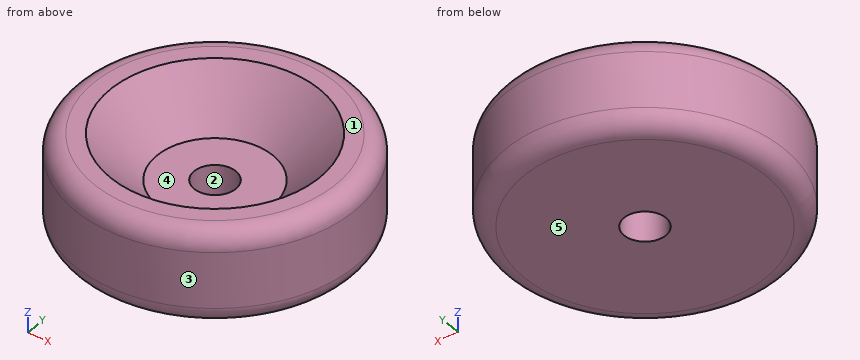
from build123d import *

# Parameters (mm, degrees)
F0_R     = 15
F0_R_2   = 11
F0_R_3   = 4.25
F1_DEPTH = 10
F2_R     = 2
F0_R_4   = 2.25
F3_DEPTH = 5


# Not quite as in the source:
# - a fillet or chamfer that OpenCascade refuses, or shapes differently, is made with other operations: its cross-section is extruded or revolved along the edge and cut away or added


with BuildPart() as f1:
    # F0 (on Top) → F1 (new body)
    with BuildSketch(Plane.XY):
        Circle(F0_R)
        Circle(F0_R_2, mode=Mode.SUBTRACT)
        Circle(F0_R_2)
        Circle(F0_R_3, mode=Mode.SUBTRACT)
    extrude(amount=F1_DEPTH)

    # F2
    f2_edges = [f1.edges().sort_by_distance(p)[0] for p in [
        (-15, 0, 10),
        (15, 0, 5),
        (-15, 0, 0),
    ]]
    fillet(f2_edges, radius=F2_R)

    # F0 (on Top) → F3 (join)
    with BuildSketch(Plane.XY):
        Circle(F0_R_3)
        Circle(F0_R_4, mode=Mode.SUBTRACT)
    extrude(amount=F3_DEPTH)

    # F4: chamfer of 7 on 1 edges, made by hand


with BuildPart() as f4_tool2:
    # F4_s3 → F4_t4 (revolve)
    with BuildSketch(Plane.XZ):
        Polygon((11.25, 10), (4.25, 3), (4.25, 10), align=None)
    revolve(axis=Axis((0, 0, 10), (0, 0, 1)))

    split(bisect_by=Plane.XY.offset(5), keep=Keep.TOP)


with BuildPart() as f1_1:
    add(f1.part)

    # F4_t1: cut F4_tool2
    add(f4_tool2.part, mode=Mode.SUBTRACT)


solid = f1_1.part
CAD build for the part. Positions are in the model's coordinates, mm. Face numbers are marked on the shaded views. A direction names the side the tool comes from. Give positions to 0.01 mm unless a question says otherwise; leave off trailing zeros. Write each loop counter-clockwise with the first axis right and the second up, starting at its lowest first coordinate (ties: lowest second). Pieces come first, ordered by that corner, then holes. Notation, with made-up numbers: (19.25, 78.5) -> (39.25, 78.5) arc R7 ccw to (39.25, 85.5) -> close; hole circle Ø11 at (57, 43). An arc over 180 degrees is marked (long way). Return JSON: item names as keys, results as strings.
Item 1: Band-saw the part on A-A (x = 0). List the corners of the cut face in (y, z).
Answer below:
{"outline": "(-15, 2) arc R2 ccw to (-13, 0) -> (-2.25, 0) -> (-2.25, 5) -> (-6.25, 5) -> (-11.25, 10) -> (-13, 10) arc R2 ccw to (-15, 8) -> close; (2.25, 0) -> (13, 0) arc R2 ccw to (15, 2) -> (15, 8) arc R2 ccw to (13, 10) -> (11.25, 10) -> (6.25, 5) -> (2.25, 5) -> close"}
Item 2: Drill centre lines: probe 1 along Y at (x, z) = (0, 2.4); probe 2 along Z at (x, y) = (-3.5, 0.5); probe 3 along Y at (x, z) = (-4.5, 8). Where is each one in solid material? Low to high.
Answer below:
{"probe 1": "y = -15 to -2.25, 2.25 to 15", "probe 2": "z = 0 to 5", "probe 3": "y = -14.31 to -8.08, 8.08 to 14.31"}
Item 3: Band-saw the part on C-C (z = 6.5). List the corners of the cut face in (x, y), then the cut area to 3 significant figures.
Answer below:
{"outline": "circle Ø30 at (0, 0); hole circle Ø15.5 at (0, 0)", "area": "518 mm2"}
Item 4: Drop flat-ended pins along their axis: pin 1 (14 mm diameter, centred on x = 1.5, y = -2, fed in from +Z); pin 2 (1 mm diameter, centred on x = 6.5, z = 1.5, fed in from -Y); pin 3 (3 mm diameter, centred on y = -7.5, z = 5.5, fed in from +X). Give the stop position or say it passes through.
Answer below:
{"pin 1": "stops at z = 8.25", "pin 2": "stops at y = -13.7", "pin 3": "stops at x = 13.75"}
Item 5: Tool access for the marked faces 4 and 5: list every direction of +Z, -Z, +X, -X, +Y, -Y with a clear straight run to the whole face (end or side of a thin tool).
Answer below:
{"face 4": "+Z", "face 5": "-Z, +X, -X, +Y, -Y"}
Item 6: Band-saw the part on D-D (z = 1). List the corners of the cut face in (x, y).
Answer below:
{"outline": "circle Ø29.46 at (0, 0); hole circle Ø4.5 at (0, 0)"}
Item 7: Two-plate mould, pull along X, no slides. Class the marked faces 1, 2 and 3: +X half, -X half, draft (parallel to the pull), parting line (faces both ways), or undercut.
Answer below:
{"face 1": "draft", "face 2": "undercut", "face 3": "parting line"}
